Part model, mm, in its own coordinate system. Coordinates: 2 decimals unless noted, no trailing zeros. Order: outer loops, then holes, each group sorted by start corner. A loop starts at its lowest first (then second) coordinate and runs counter-clockwise, first axis right, second up.
1) Wall check: L1, parallel to X at y = 11, z = 3; L2, parallel to Y at x = 9, z = 1.25; L3, parallel to Y at x = 49.5, z = 2.5. Give the ranges that are in metal, low to high.
2) Cut at A-A (z = 5.75). List the corners of the cut face in (x, y) (3 decimals), and give its area (3 significant figures).
3) Cut at C-C (z = 3). List the corners of the cut face in (x, y) (3 decimals).
4) Mould opens along Y. For faces 1 (the flat face through (30, 0, 6)), 2 (the flat face through (60.312, 9, 8)), 3 (the cylindrical face through (4.244, 10.866, 6.399)), 4 (the cylindrical face through (56.068, 10.866, 6.047)) say: +Y half, -Y half, draft (parallel to the pull), parting line (faces both ways), or undercut.
5) Cut at B-B (x = 55). List the corners of the cut face in (y, z) (3 decimals).
6) Pin check, flat tips, straight feed: pin 1 Ø2.5 at (y, z) = (9.525, 6.223) entering from +X; pin 2 Ø1.6 at (y, z) = (9.525, 6.223) entering from +X; pin 3 Ø3 at (x, y) = (9.525, 9.525) entering from +Z. Stop position of each tip, or through.
```python
from build123d import *

# Parameters (mm, degrees)
SKETCH1_W                 = 60.3123
SKETCH1_H                 = 19.05
EXTRUDE1_DEPTH            = 12.573
SKETCH2_R                 = 1.778
CUT_EXTRUDE1_DEPTH        = 13.573
F_6_32_TAPPED_HOLE1_D     = 2.7051
F_6_32_TAPPED_HOLE1_DEPTH = 9.525
F_6_32_TAPPED_HOLE1_TIP   = 0.81269403
F_6_32_TAPPED_HOLE2_D     = 2.7051
F_6_32_TAPPED_HOLE2_DEPTH = 9.525
F_6_32_TAPPED_HOLE2_TIP   = 0.81269403


with BuildPart() as part:
    # Sketch1 → Extrude1 (new body)
    with BuildSketch(Plane.XY):
        with Locations((30.15615, 9.525)):
            Rectangle(SKETCH1_W, SKETCH1_H)
    extrude(amount=EXTRUDE1_DEPTH)

    # Sketch2 → Cut-Extrude1 (cut, through all)
    with BuildSketch(Plane.XY.offset(12.573)):
        with Locations((9.525, 9.525)):
            Circle(SKETCH2_R)
        with Locations((50.7873, 9.525)):
            Circle(SKETCH2_R)
    extrude(amount=-CUT_EXTRUDE1_DEPTH, mode=Mode.SUBTRACT)

    # #6-32 Tapped Hole1
    with Locations(Plane.ZY):
        with Locations((6.223, 9.525)):
            Hole(F_6_32_TAPPED_HOLE1_D / 2, depth=F_6_32_TAPPED_HOLE1_DEPTH)
            with Locations((0, 0, -(F_6_32_TAPPED_HOLE1_DEPTH + F_6_32_TAPPED_HOLE1_TIP / 2))):  # 118° drill point
                Cone(0, F_6_32_TAPPED_HOLE1_D / 2, F_6_32_TAPPED_HOLE1_TIP, mode=Mode.SUBTRACT)

    # #6-32 Tapped Hole2
    with Locations(Plane(origin=(60.3123, 0, 0), x_dir=(0, 0, -1), z_dir=(1, 0, 0))):
        with Locations((-6.223, 9.525)):
            Hole(F_6_32_TAPPED_HOLE2_D / 2, depth=F_6_32_TAPPED_HOLE2_DEPTH)
            with Locations((0, 0, -(F_6_32_TAPPED_HOLE2_DEPTH + F_6_32_TAPPED_HOLE2_TIP / 2))):  # 118° drill point
                Cone(0, F_6_32_TAPPED_HOLE2_D / 2, F_6_32_TAPPED_HOLE2_TIP, mode=Mode.SUBTRACT)


solid = part.part
```
Geometry check:
1. L1: x = 0 to 8.53, 10.52 to 49.79, 51.78 to 60.31
1. L2: y = 0 to 7.83, 11.22 to 19.05
1. L3: y = 0 to 8.3, 10.75 to 19.05
2. outline: (0, 0) - (60.312, 0) - (60.312, 8.258) - (52.035, 8.258) arc R1.778 cw (long way) to (52.035, 10.792) - (60.312, 10.792) - (60.312, 19.05) - (0, 19.05) - (0, 10.792) - (8.278, 10.792) arc R1.778 cw (long way) to (8.278, 8.258) - (0, 8.258) - close
2. area: 1,090 mm2
3. outline: (0, 0) - (60.312, 0) - (60.312, 19.05) - (0, 19.05) - close; hole circle Ø3.556 at (9.525, 9.525); hole circle Ø3.556 at (50.787, 9.525)
4. face 1: -Y half
4. face 2: draft
4. face 3: undercut
4. face 4: undercut
5. outline: (0, 0) - (19.05, 0) - (19.05, 12.573) - (0, 12.573) - close; hole circle Ø2.705 at (9.525, 6.223)
6. pin 1: stops at x = 49.52
6. pin 2: stops at x = 49.2
6. pin 3: passes through
